from build123d import *

# Parameters (mm, degrees)
AUFSATZ_LINEAR_AUSTRAGEN1_DEPTH           = 2
F_1_2_1_2_DURCHMESSER_BOHRUNG1_AT_2_COUNT = 2
F_1_2_1_2_DURCHMESSER_BOHRUNG1_AT_2_PITCH = 6
F_1_2_1_2_DURCHMESSER_BOHRUNG1_AT_3_COUNT = 2
F_1_2_1_2_DURCHMESSER_BOHRUNG1_AT_3_PITCH = 9
F_1_2_1_2_DURCHMESSER_BOHRUNG1_AT_4_COUNT = 2
F_1_2_1_2_DURCHMESSER_BOHRUNG1_AT_4_PITCH = 3
F_1_2_1_2_DURCHMESSER_BOHRUNG1_AT_5_COUNT = 2
F_1_2_1_2_DURCHMESSER_BOHRUNG1_AT_5_PITCH = 23.546655814
F_1_2_1_2_DURCHMESSER_BOHRUNG1_AT_6_COUNT = 2
F_1_2_1_2_DURCHMESSER_BOHRUNG1_AT_6_PITCH = 21.530095216
F_1_2_1_2_DURCHMESSER_BOHRUNG1_AT_7_COUNT = 2
F_1_2_1_2_DURCHMESSER_BOHRUNG1_AT_7_PITCH = 19.764741334
F_1_2_1_2_DURCHMESSER_BOHRUNG1_AT_8_COUNT = 2
F_1_2_1_2_DURCHMESSER_BOHRUNG1_AT_8_PITCH = 18.323345764
SKIZZE4_W                                 = 0.7
SKIZZE4_H                                 = 0.5
F_2_9_2_9_DURCHMESSER_BOHRUNG1_D          = 2.9
F_2_7_2_7_DIAMETER_HOLE1_D                = 2.7
F_2_7_2_7_DIAMETER_HOLE1_DEPTH            = 2.7


with BuildPart() as part:
    # Skizze1 → Aufsatz-Linear austragen1 (new body)
    with BuildSketch(Plane.XY):
        with BuildLine():
            Line((-2.30327731, 17.116276346), (-4.25, 7.5))
            ThreePointArc((-4.25, 7.5), (-4.666990822, 4.666990822), (-7.5, 4.25))
            Line((-7.5, 4.25), (-17.116276346, 2.30327731))
            ThreePointArc((-17.116276346, 2.30327731), (-19, 0), (-17.116276346, -2.30327731))
            Line((-17.116276346, -2.30327731), (-7.5, -4.25))
            ThreePointArc((-7.5, -4.25), (-4.666990822, -4.666990822), (-4.25, -7.5))
            Line((-4.25, -7.5), (-2.30327731, -17.116276346))
            ThreePointArc((-2.30327731, -17.116276346), (0, -19), (2.30327731, -17.116276346))
            Line((2.30327731, -17.116276346), (4.25, -7.5))
            ThreePointArc((4.25, -7.5), (4.666990822, -4.666990822), (7.5, -4.25))
            Line((7.5, -4.25), (17.116276346, -2.30327731))
            ThreePointArc((17.116276346, -2.30327731), (19, 0), (17.116276346, 2.30327731))
            Line((17.116276346, 2.30327731), (7.5, 4.25))
            ThreePointArc((7.5, 4.25), (4.666990822, 4.666990822), (4.25, 7.5))
            Line((4.25, 7.5), (2.30327731, 17.116276346))
            ThreePointArc((2.30327731, 17.116276346), (0, 19), (-2.30327731, 17.116276346))
        make_face()
    extrude(amount=AUFSATZ_LINEAR_AUSTRAGEN1_DEPTH)

    # Skizze2 → Ø1.2 (1.2) Durchmesser Bohrung1 (revolve, cut)
    with BuildSketch(Plane(origin=(0, 16.65, 0), x_dir=(0, 1, 0), z_dir=(1, 0, 0))):
        Polygon((0, 0), (0, 10.360516371), (0.6, 10), (0.6, 0), align=None)
    f_1_2_1_2_durchmesser_bohrung1 = revolve(axis=Axis((0, 16.65, -6.35), (0, 0, 1)), mode=Mode.SUBTRACT)

    # Ø1.2 (1.2) Durchmesser Bohrung1 at 2: Ø1.2 (1.2) Durchmesser Bohrung1 ×2
    with Locations(*[(0, -i * F_1_2_1_2_DURCHMESSER_BOHRUNG1_AT_2_PITCH, 0) for i in range(1, F_1_2_1_2_DURCHMESSER_BOHRUNG1_AT_2_COUNT)]):
        add(f_1_2_1_2_durchmesser_bohrung1, mode=Mode.SUBTRACT)

    # Ø1.2 (1.2) Durchmesser Bohrung1 at 3: Ø1.2 (1.2) Durchmesser Bohrung1 ×2
    with Locations(*[(0, -i * F_1_2_1_2_DURCHMESSER_BOHRUNG1_AT_3_PITCH, 0) for i in range(1, F_1_2_1_2_DURCHMESSER_BOHRUNG1_AT_3_COUNT)]):
        add(f_1_2_1_2_durchmesser_bohrung1, mode=Mode.SUBTRACT)

    # Ø1.2 (1.2) Durchmesser Bohrung1 at 4: Ø1.2 (1.2) Durchmesser Bohrung1 ×2
    with Locations(*[(0, -i * F_1_2_1_2_DURCHMESSER_BOHRUNG1_AT_4_PITCH, 0) for i in range(1, F_1_2_1_2_DURCHMESSER_BOHRUNG1_AT_4_COUNT)]):
        add(f_1_2_1_2_durchmesser_bohrung1, mode=Mode.SUBTRACT)

    # Ø1.2 (1.2) Durchmesser Bohrung1 at 5: Ø1.2 (1.2) Durchmesser Bohrung1 ×2
    with Locations(*[Vector(-0.707106781, -0.707106781, 0) * (i * F_1_2_1_2_DURCHMESSER_BOHRUNG1_AT_5_PITCH) for i in range(1, F_1_2_1_2_DURCHMESSER_BOHRUNG1_AT_5_COUNT)]):
        add(f_1_2_1_2_durchmesser_bohrung1, mode=Mode.SUBTRACT)

    # Ø1.2 (1.2) Durchmesser Bohrung1 at 6: Ø1.2 (1.2) Durchmesser Bohrung1 ×2
    with Locations(*[Vector(-0.633996267, -0.773336106, 0) * (i * F_1_2_1_2_DURCHMESSER_BOHRUNG1_AT_6_PITCH) for i in range(1, F_1_2_1_2_DURCHMESSER_BOHRUNG1_AT_6_COUNT)]):
        add(f_1_2_1_2_durchmesser_bohrung1, mode=Mode.SUBTRACT)

    # Ø1.2 (1.2) Durchmesser Bohrung1 at 7: Ø1.2 (1.2) Durchmesser Bohrung1 ×2
    with Locations(*[Vector(-0.538838319, -0.842409203, 0) * (i * F_1_2_1_2_DURCHMESSER_BOHRUNG1_AT_7_PITCH) for i in range(1, F_1_2_1_2_DURCHMESSER_BOHRUNG1_AT_7_COUNT)]):
        add(f_1_2_1_2_durchmesser_bohrung1, mode=Mode.SUBTRACT)

    # Ø1.2 (1.2) Durchmesser Bohrung1 at 8: Ø1.2 (1.2) Durchmesser Bohrung1 ×2
    with Locations(*[Vector(-0.417500172, -0.908676844, 0) * (i * F_1_2_1_2_DURCHMESSER_BOHRUNG1_AT_8_PITCH) for i in range(1, F_1_2_1_2_DURCHMESSER_BOHRUNG1_AT_8_COUNT)]):
        add(f_1_2_1_2_durchmesser_bohrung1, mode=Mode.SUBTRACT)

    # Spiegeln1: Ø1.2 (1.2) Durchmesser Bohrung1 across plane
    add(f_1_2_1_2_durchmesser_bohrung1.mirror(Plane(origin=(0, 0, 0), x_dir=(0, 0, 1), z_dir=(1, 0, 0))), mode=Mode.SUBTRACT)

    # Spiegeln1 copy 1 sketch → Spiegeln1 copy 1 (revolve, cut)
    with BuildSketch(Plane(origin=(0, 10.65, 0), x_dir=(0, 1, 0), z_dir=(-1, 0, 0))):
        Polygon((0, 0), (0, -10.360516371), (0.6, -10), (0.6, 0), align=None)
    revolve(axis=Axis((0, 10.65, -6.35), (0, 0, -1)), mode=Mode.SUBTRACT)

    # Spiegeln1 copy 2 sketch → Spiegeln1 copy 2 (revolve, cut)
    with BuildSketch(Plane(origin=(0, 7.65, 0), x_dir=(0, 1, 0), z_dir=(-1, 0, 0))):
        Polygon((0, 0), (0, -10.360516371), (0.6, -10), (0.6, 0), align=None)
    revolve(axis=Axis((0, 7.65, -6.35), (0, 0, -1)), mode=Mode.SUBTRACT)

    # Spiegeln1 copy 3 sketch → Spiegeln1 copy 3 (revolve, cut)
    with BuildSketch(Plane(origin=(0, 13.65, 0), x_dir=(0, 1, 0), z_dir=(-1, 0, 0))):
        Polygon((0, 0), (0, -10.360516371), (0.6, -10), (0.6, 0), align=None)
    revolve(axis=Axis((0, 13.65, -6.35), (0, 0, -1)), mode=Mode.SUBTRACT)

    # Spiegeln1 copy 4 sketch → Spiegeln1 copy 4 (revolve, cut)
    with BuildSketch(Plane(origin=(16.65, 0, 0), x_dir=(0, 1, 0), z_dir=(-1, 0, 0))):
        Polygon((0, 0), (0, -10.360516371), (0.6, -10), (0.6, 0), align=None)
    revolve(axis=Axis((16.65, 0, -6.35), (0, 0, -1)), mode=Mode.SUBTRACT)

    # Spiegeln1 copy 5 sketch → Spiegeln1 copy 5 (revolve, cut)
    with BuildSketch(Plane(origin=(13.65, 0, 0), x_dir=(0, 1, 0), z_dir=(-1, 0, 0))):
        Polygon((0, 0), (0, -10.360516371), (0.6, -10), (0.6, 0), align=None)
    revolve(axis=Axis((13.65, 0, -6.35), (0, 0, -1)), mode=Mode.SUBTRACT)

    # Spiegeln1 copy 6 sketch → Spiegeln1 copy 6 (revolve, cut)
    with BuildSketch(Plane(origin=(10.65, 0, 0), x_dir=(0, 1, 0), z_dir=(-1, 0, 0))):
        Polygon((0, 0), (0, -10.360516371), (0.6, -10), (0.6, 0), align=None)
    revolve(axis=Axis((10.65, 0, -6.35), (0, 0, -1)), mode=Mode.SUBTRACT)

    # Spiegeln1 copy 7 sketch → Spiegeln1 copy 7 (revolve, cut)
    with BuildSketch(Plane(origin=(7.65, 0, 0), x_dir=(0, 1, 0), z_dir=(-1, 0, 0))):
        Polygon((0, 0), (0, -10.360516371), (0.6, -10), (0.6, 0), align=None)
    revolve(axis=Axis((7.65, 0, -6.35), (0, 0, -1)), mode=Mode.SUBTRACT)

    # Spiegeln2: Ø1.2 (1.2) Durchmesser Bohrung1 across plane
    add(f_1_2_1_2_durchmesser_bohrung1.mirror(Plane.ZX), mode=Mode.SUBTRACT)

    # Spiegeln2 copy 1 sketch → Spiegeln2 copy 1 (revolve, cut)
    with BuildSketch(Plane(origin=(0, -10.65, 0), x_dir=(0, -1, 0), z_dir=(1, 0, 0))):
        Polygon((0, 0), (0, -10.360516371), (0.6, -10), (0.6, 0), align=None)
    revolve(axis=Axis((0, -10.65, -6.35), (0, 0, -1)), mode=Mode.SUBTRACT)

    # Spiegeln2 copy 2 sketch → Spiegeln2 copy 2 (revolve, cut)
    with BuildSketch(Plane(origin=(0, -7.65, 0), x_dir=(0, -1, 0), z_dir=(1, 0, 0))):
        Polygon((0, 0), (0, -10.360516371), (0.6, -10), (0.6, 0), align=None)
    revolve(axis=Axis((0, -7.65, -6.35), (0, 0, -1)), mode=Mode.SUBTRACT)

    # Spiegeln2 copy 3 sketch → Spiegeln2 copy 3 (revolve, cut)
    with BuildSketch(Plane(origin=(0, -13.65, 0), x_dir=(0, -1, 0), z_dir=(1, 0, 0))):
        Polygon((0, 0), (0, -10.360516371), (0.6, -10), (0.6, 0), align=None)
    revolve(axis=Axis((0, -13.65, -6.35), (0, 0, -1)), mode=Mode.SUBTRACT)

    # Spiegeln2 copy 4 sketch → Spiegeln2 copy 4 (revolve, cut)
    with BuildSketch(Plane(origin=(-16.65, 0, 0), x_dir=(0, -1, 0), z_dir=(1, 0, 0))):
        Polygon((0, 0), (0, -10.360516371), (0.6, -10), (0.6, 0), align=None)
    revolve(axis=Axis((-16.65, 0, -6.35), (0, 0, -1)), mode=Mode.SUBTRACT)

    # Spiegeln2 copy 5 sketch → Spiegeln2 copy 5 (revolve, cut)
    with BuildSketch(Plane(origin=(-13.65, 0, 0), x_dir=(0, -1, 0), z_dir=(1, 0, 0))):
        Polygon((0, 0), (0, -10.360516371), (0.6, -10), (0.6, 0), align=None)
    revolve(axis=Axis((-13.65, 0, -6.35), (0, 0, -1)), mode=Mode.SUBTRACT)

    # Spiegeln2 copy 6 sketch → Spiegeln2 copy 6 (revolve, cut)
    with BuildSketch(Plane(origin=(-10.65, 0, 0), x_dir=(0, -1, 0), z_dir=(1, 0, 0))):
        Polygon((0, 0), (0, -10.360516371), (0.6, -10), (0.6, 0), align=None)
    revolve(axis=Axis((-10.65, 0, -6.35), (0, 0, -1)), mode=Mode.SUBTRACT)

    # Spiegeln2 copy 7 sketch → Spiegeln2 copy 7 (revolve, cut)
    with BuildSketch(Plane(origin=(-7.65, 0, 0), x_dir=(0, -1, 0), z_dir=(1, 0, 0))):
        Polygon((0, 0), (0, -10.360516371), (0.6, -10), (0.6, 0), align=None)
    revolve(axis=Axis((-7.65, 0, -6.35), (0, 0, -1)), mode=Mode.SUBTRACT)

    # Skizze4 → Rotation1 (revolve)
    with BuildSketch(Plane(origin=(0, 0, 0), x_dir=(0, 0, -1), z_dir=(1, 0, 0))):
        with BuildLine():
            Line((0, 5), (1, 5))
            ThreePointArc((1, 5), (1.439339828, 3.939339828), (2.5, 3.5))
            Line((2.5, 3.5), (3.5, 3.5))
            Line((3.5, 3.5), (3.5, 3))
            Line((3.5, 3), (0, 3))
            Line((0, 3), (0, 5))
        make_face()
        with Locations((-2.35, 3.25)):
            Rectangle(SKIZZE4_W, SKIZZE4_H)
    revolve(axis=Axis((0, 0, 3.110475716), (0, 0, -1)))

    # Ø2.9 (2.9) Durchmesser Bohrung1 (through all)
    with Locations(Plane(origin=(0, 0, 0), x_dir=(-1, 0, 0), z_dir=(0, 0, -1))):
        with Locations((0, 0)):
            Hole(F_2_9_2_9_DURCHMESSER_BOHRUNG1_D / 2)

    # Ø2.7 (2.7) Diameter Hole1
    with Locations(Plane(origin=(0, 0, 0), x_dir=(-1, 0, 0), z_dir=(0, 0, -1))):
        with Locations((-7.65, 0), (7.65, 0), (0, 10.65), (0, -10.65)):
            Hole(F_2_7_2_7_DIAMETER_HOLE1_D / 2, depth=F_2_7_2_7_DIAMETER_HOLE1_DEPTH)


solid = part.part
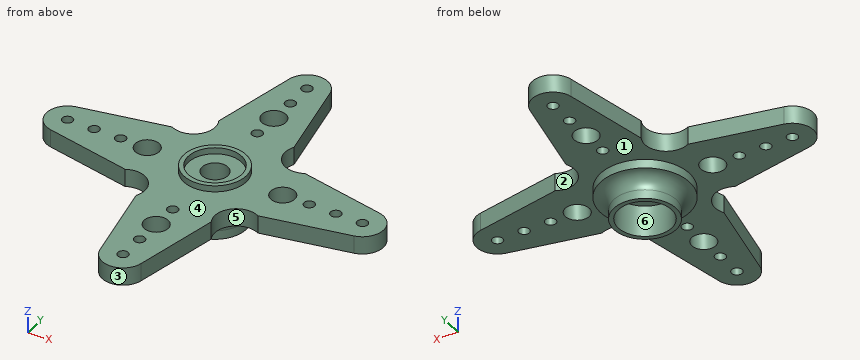
Could you check a few things on this model? Use its own coordinates, in mm. Face numbers are marked on the shaded views. A direction names the side the tool comes from. Give positions to 0.01 mm unless a question says otherwise; leave off trailing zeros. Write each loop counter-clockwise with the first axis right and the second up, starting at its lowest first coordinate (ties: lowest second). Pieces come first, ordered by that corner, then holes. Notation, with made-up numbers: (64.25, 58.5) - (101.25, 58.5) arc R13 ccw to (101.25, 64.5) - close; hole circle Ø5 at (-24, 48). An arc over 180 degrees is marked (long way). Use CSV: the item, a comma, the result in double quotes. Start each with the question number.
Item 1: I want a section at C-C, the plane x = -10.65. Please give me the cut outline in (y, z).
Item 2: If we mould it in two halves opening along X, with no side actions, what happens to the marked faces 1, 2 and 3? For each: pulls with the +X half, pulls with the -X half, needs draft (parallel to the pull), parting line crosses it, or undercut.
Item 3: I want a section at D-D, the plane x = 12. Please give me the cut outline in (y, z).
Item 4: I'm going to push flat-ended pins straight in: pin 1 (8 mm diameter, centred on x = 0, y = 0, fed in from +Z); pin 2 (1.9 mm diameter, centred on x = -16.65, y = 0, fed in from +Z); pin 3 (1 mm diameter, centred on x = -5, y = 9.5, fed in from -Z); pin 4 (1.5 mm diameter, centred on x = 6.5, z = 1.5, fed in from +Y). Where does each tip first touch, or does it pass through?
Item 5: For the marked faces 4, 5 and 6, which set-ups out of +Z, -Z, +X, -X, +Y, -Y let a thin tool reach every point of the face, with its end or its side?
Item 6: I want a section at A-A, the plane y = -10.65. Please give me the cut outline in (x, z), then the cut area to 3 significant figures.
Item 7: I want a section at B-B, the plane z = 1. Give the number of separate pieces and of enclosed holes in the cut face, then the cut area to 3 significant figures.
Item 8: If I drill on line 1 along X through (y, z) = (13.65, 0.8) (3 decimals); line 2 along Z through (x, y) = (-3, -9); line 3 along X through (y, z) = (-17, 1), over which ranges is the centre line in solid material (lowest first)?
Findings:
1,outline,"(-3.61, 0) - (-0.6, 0) - (-0.6, 2) - (-3.61, 2) - close; (0.6, 0) - (3.61, 0) - (3.61, 2) - (0.6, 2) - close"
2,face 1,"needs draft"
2,face 2,"undercut"
2,face 3,"parting line crosses it"
3,outline,"(-3.34, 0) - (3.34, 0) - (3.34, 2) - (-3.34, 2) - close"
4,pin 1,"stops at z = 2.7"
4,pin 2,"stops at z = 2"
4,pin 3,"passes through"
4,pin 4,"stops at y = 4.13"
5,face 4,"+Z"
5,face 5,"+Z, -Z"
5,face 6,"-Z"
6,outline,"(-3.61, 0) - (-1.35, 0) - (-1.35, 2) - (-3.61, 2) - close; (1.35, 0) - (3.61, 0) - (3.61, 2) - (1.35, 2) - close"
6,area,"9.05 mm2"
7,separate pieces,"1"
7,enclosed holes,"17"
7,area,"416 mm2"
8,line 1,"x = -3.005 to -0.6, 0.6 to 3.005"
8,line 2,"z = 0 to 2"
8,line 3,"x = -2.33 to -0.49, 0.49 to 2.33"
